from build123d import *

# Parameters (mm, degrees)
SKETCH1_W           = 50
SKETCH1_H           = 140
BOSS_EXTRUDE1_DEPTH = 15
SKETCH1_3_R         = 7.5
CUT_EXTRUDE1_DEPTH  = 76.828754441
FILLET1_R           = 15


with BuildPart() as part:
    # Sketch1 → Boss-Extrude1 (new body)
    with BuildSketch(Plane(origin=(0, 0, 0), x_dir=(0, 0, -1), z_dir=(1, 0, 0))):
        Rectangle(SKETCH1_W, SKETCH1_H)
    extrude(amount=BOSS_EXTRUDE1_DEPTH)

    # Sketch1<3> → Cut-Extrude1 (cut, through all)
    with BuildSketch(Plane(origin=(0, 0, 0), x_dir=(0, 0, -1), z_dir=(1, 0, 0))):
        with Locations((0, 50)):
            Circle(SKETCH1_3_R)
        with Locations((0, -50)):
            Circle(SKETCH1_3_R)
    extrude(amount=CUT_EXTRUDE1_DEPTH, mode=Mode.SUBTRACT)

    # Fillet1
    fillet1_edges = [part.edges().sort_by_distance(p)[0] for p in [
        (7.5, -70, -25),
        (7.5, -70, 25),
        (7.5, 70, 25),
        (7.5, 70, -25),
    ]]
    fillet(fillet1_edges, radius=FILLET1_R)


solid = part.part
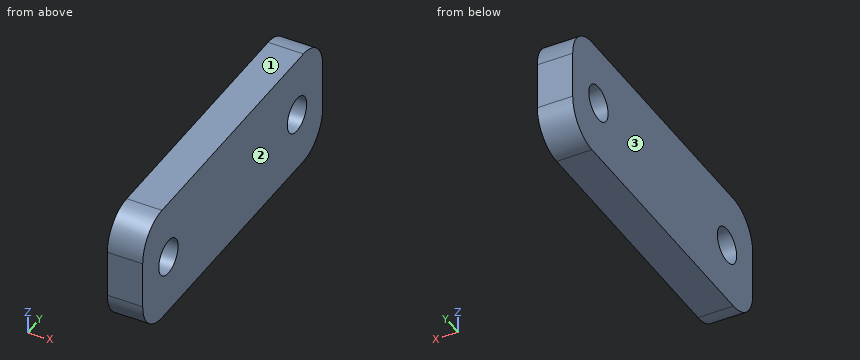
Part model, mm, in its own coordinate system. Face numbers are marked on the shaded views. Give positions to 0.01 mm unless a question says otherwise; leave off trailing zeros. Write each loop counter-clockwise with the first axis right and the second up, starting at its lowest first coordinate (ties: lowest second). Pieces come first, ordered by that corner, then holes.
1) Two-plate mould, pull along X, no slides. Class the marked faces 1, 2 and 3: released by +X, released by -X, zero draft, split by the parting line, or undercut.
Resolved:
face 1: zero draft
face 2: released by +X
face 3: released by -X
2) Cut at A-A on y = -50. Write the cut outline in (x, z), then the cut area to 3 significant figures.
Resolved:
outline: (0, -25) - (15, -25) - (15, -7.5) - (0, -7.5) - close; (0, 7.5) - (15, 7.5) - (15, 25) - (0, 25) - close
area: 525 mm2
3) Cut at B-B on z = 0. Write the cut outline in (x, y).
Resolved:
outline: (0, -70) - (15, -70) - (15, -57.5) - (0, -57.5) - close; (0, -42.5) - (15, -42.5) - (15, 42.5) - (0, 42.5) - close; (0, 57.5) - (15, 57.5) - (15, 70) - (0, 70) - close
4) Cut at D-D on z = -6. Write the cut outline in (x, y), then the cut area to 3 significant figures.
Resolved:
outline: (0, -70) - (15, -70) - (15, -54.5) - (0, -54.5) - close; (0, -45.5) - (15, -45.5) - (15, 45.5) - (0, 45.5) - close; (0, 54.5) - (15, 54.5) - (15, 70) - (0, 70) - close
area: 1,830 mm2
5) Probe L1, parallel to Y at x = 8.75, z = 0; L2, parallel to Z at x = 3.75, y = -50; L3, parallel to Y at x = 13.75, z = 2.5. List the from-to ranges inside material, lowest first.
Resolved:
L1: y = -70 to -57.5, -42.5 to 42.5, 57.5 to 70
L2: z = -25 to -7.5, 7.5 to 25
L3: y = -70 to -57.07, -42.93 to 42.93, 57.07 to 70
6) Cut at C-C on x = 8. Write the cut outline in (y, z).
Resolved:
outline: (-70, -10) arc R15 ccw to (-55, -25) - (55, -25) arc R15 ccw to (70, -10) - (70, 10) arc R15 ccw to (55, 25) - (-55, 25) arc R15 ccw to (-70, 10) - close; hole circle Ø15 at (-50, 0); hole circle Ø15 at (50, 0)
